Design review of the part built by this model. Coordinates are the model's own, in mm. Face numbers are marked on the shaded views. A direction names the side the tool comes from. Give positions to 0.01 mm unless a question says otherwise; leave off trailing zeros. Loops run counter-clockwise (first coordinate to the right, second up) from the corner with the lowest first, then second, coordinate; pieces in that order, holes last. Notation, with made-up numbers: (61, -17) -> (100, -17) arc R21 ccw to (100, 10) -> close; hole circle Ø4 at (-15.5, 20.25). An arc over 180 degrees is marked (long way). Answer as CSV lines item,"result".
from build123d import *

# Parameters (mm, degrees)
SKETCH_1_R          = 1.95
EXTRUDE_1_DEPTH     = 19
SKETCH_4_W          = 2
SKETCH_4_H          = 9
EXTRUDE_2_DEPTH     = 1.95
CUT_EXTRUDE_1_DEPTH = 21.359396
EXTRUDE_4_DEPTH     = 15.9
SKETCH_9_R          = 2
CUT_EXTRUDE_2_DEPTH = 17
SKETCH_11_R         = 3
CUT_EXTRUDE_4_DEPTH = 0.5


with BuildPart() as part:
    # 스케치1 → 보스-돌출1 (new body)
    with BuildSketch(Plane.XY):
        Circle(SKETCH_1_R)
    extrude(amount=EXTRUDE_1_DEPTH)

    # 스케치4 → 보스-돌출2 (add, symmetric)
    with BuildSketch(Plane(origin=(0, 0, 0), x_dir=(0, 0, -1), z_dir=(1, 0, 0))):
        with Locations((-1, -2.55)):
            Rectangle(SKETCH_4_W, SKETCH_4_H)
    extrude(amount=EXTRUDE_2_DEPTH, both=True)

    # 스케치5 → 컷-돌출1 (cut, through all)
    with BuildSketch(Plane.XY.offset(19)):
        with BuildLine():
            Line((-1.95, 1.95), (-1.95, 0))
            ThreePointArc((-1.95, 0), (-1.378858, 1.378858), (0, 1.95))
            Line((0, 1.95), (-1.95, 1.95))
        make_face()
        with BuildLine():
            ThreePointArc((0, 1.95), (1.378858, 1.378858), (1.95, 0))
            Line((1.95, 0), (1.95, 1.95))
            Line((1.95, 1.95), (0, 1.95))
        make_face()
    extrude(amount=-CUT_EXTRUDE_1_DEPTH, mode=Mode.SUBTRACT)

    # 스케치8 → 보스-돌출4 (add)
    with BuildSketch(Plane.XY.offset(2)):
        with BuildLine():
            ThreePointArc((1.95, -2.279803), (0, -3), (-1.95, -2.279803))
            Line((-1.95, -2.279803), (-1.95, -7.05))
            Line((-1.95, -7.05), (1.95, -7.05))
            Line((1.95, -7.05), (1.95, -2.279803))
        make_face()
    extrude(amount=EXTRUDE_4_DEPTH)

    # 스케치9 → 컷-돌출2 (cut)
    with BuildSketch(Plane.ZY.offset(1.95)):
        with Locations((9, -7.55)):
            Circle(SKETCH_9_R)
    extrude(amount=-CUT_EXTRUDE_2_DEPTH, mode=Mode.SUBTRACT)

    # 스케치11 → 컷-돌출4 (cut)
    with BuildSketch(Plane(origin=(1.95, 0, 0), x_dir=(0, 0, -1), z_dir=(1, 0, 0))):
        with Locations((-9.176059, -7.55)):
            Circle(SKETCH_11_R)
    extrude(amount=-CUT_EXTRUDE_4_DEPTH, mode=Mode.SUBTRACT)


solid = part.part
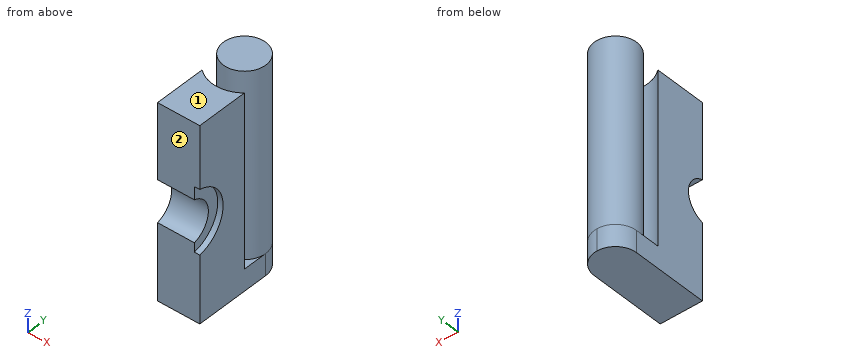
Q1. We need section B-B, the plane x = -1.2. State the section outline as (y, z) points.
Filled sheet:
outline,"(-7.05, 0) -> (1.54, 0) -> (1.54, 19) -> (-1.54, 19) -> (-1.54, 2) -> (-2.75, 2) -> (-2.75, 17.9) -> (-7.05, 17.9) -> (-7.05, 10.94) arc R2 cw to (-7.05, 7.06) -> close"
Q2. Clearance check with flat-ended pins moving along their axes: pin 1 Ø1.3 at (y, z) = (-6, 10) entering from +X; pin 2 Ø2 at (x, y) = (-1.5, -3.5) entering from +Z. State where each tip first meets the part, or that it passes through.
Filled sheet:
pin 1,"stops at x = 1.45"
pin 2,"stops at z = 17.9"
Q3. We need section A-A, the plane z = 7.5. State the section outline as (x, y) points.
Filled sheet:
outline,"(-1.95, -6.23) -> (1.45, -6.23) -> (1.45, -5.06) -> (1.95, -5.06) -> (1.95, -2.28) arc R3 cw to (-1.95, -2.28) -> close; circle Ø3.9 at (0, 0)"
Q4. We need section D-D, the plane z = 4. State the section outline as (x, y) points.
Filled sheet:
outline,"(-1.95, -7.05) -> (1.95, -7.05) -> (1.95, -2.28) arc R3 cw to (-1.95, -2.28) -> close; circle Ø3.9 at (0, 0)"
Q5. We need section C-C, the plane y = -1.75. State the section outline as (x, z) points, and give its area (3 significant figures).
Filled sheet:
outline,"(-1.95, 0) -> (1.95, 0) -> (1.95, 2) -> (0.86, 2) -> (0.86, 19) -> (-0.86, 19) -> (-0.86, 2) -> (-1.95, 2) -> close"
area,"37.0 mm^2"
Q6. For the marked faces 1 and 2, list the 3-axis set-ups (+Z, -Z, +X, -X, +Y, -Y) from which the entire face can be reached by the end or side of a thin tool; tool diameter is ignored.
Filled sheet:
face 1,"+Z, +X, -X, -Y"
face 2,"+Z, -Z, +X, -X, -Y"
Q7. To check wall thickness, follow probe 1 along X at (y, z) = (-5, 9); probe 2 along Z at (x, y) = (1.1, -3.5); probe 3 along Y at (x, z) = (-0.2, 2.75). State the ranges of each line that lie inside material, in increasing order. Write a range as from..to.
Filled sheet:
probe 1,"x = -1.95..1.45"
probe 2,"z = 0..17.9"
probe 3,"y = -7.05..-2.99, -1.94..1.94"
